Study the drawing (mm; zero at the part's minimum x, y, z) and answer. Coordinates: 2 decimals unless noted, no trailing zeros. Order: outer loops, then holes, each group sorted by start corner. A loop starts at its lowest first (then second) coordinate and runs counter-clockwise, first axis right, second up.
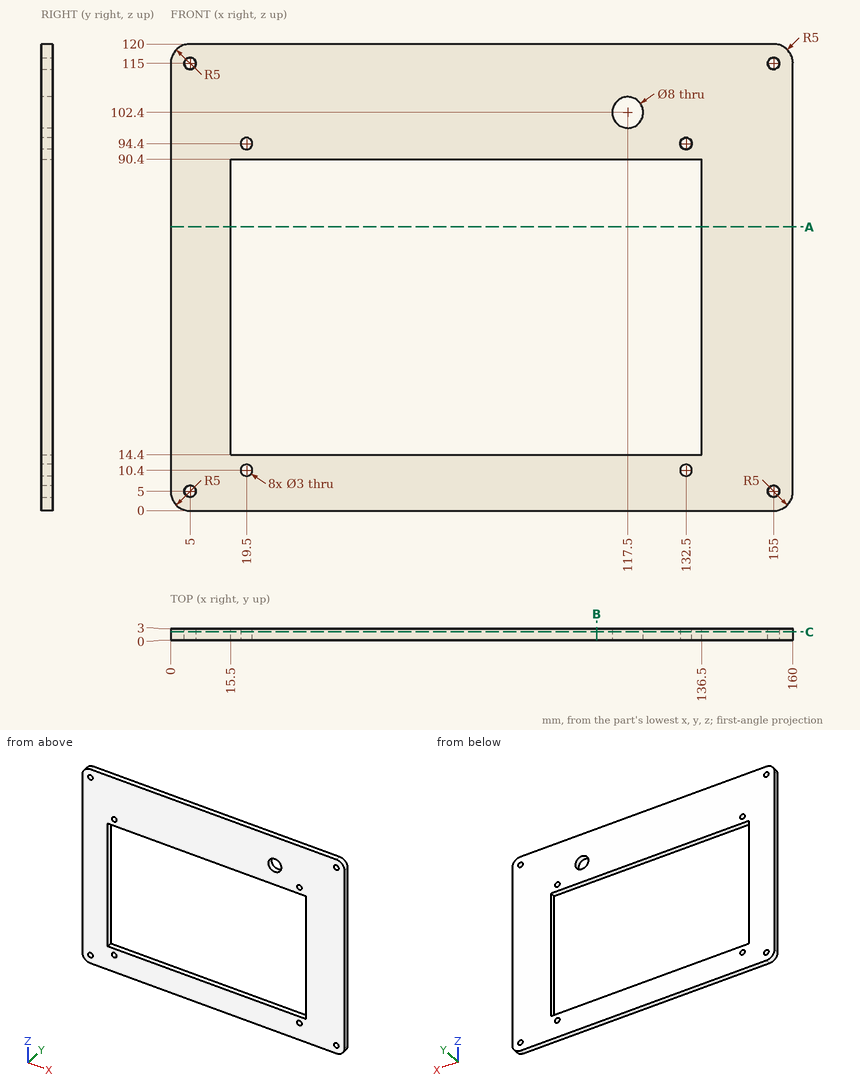
1) A cutting plane is placed at A-A, the plane z = 73. Determine the outline of the cut face in (x, y), and give its area (3 significant figures).
A:
outline: (0, 0) - (15.5, 0) - (15.5, 3) - (0, 3) - close; (136.5, 0) - (160, 0) - (160, 3) - (136.5, 3) - close
area: 117 mm2
2) A cutting plane is placed at C-C, the plane y = 2.2. State how many separate pieces and enclosed holes the cut face has, and give its area (3 significant figures).
A:
separate pieces: 1
enclosed holes: 10
area: 9,880 mm2
3) Straight lines are drawn through the part: line 1 (Z direction, x = 19.5, y = 0.8); line 2 (X direction, y = 1, z = 5); line 3 (Z direction, x = 35, y = 2.05). For each, find the intervals that lie inside material, in ascending order.
A:
line 1: z = 0 to 8.9, 11.9 to 14.4, 90.4 to 92.9, 95.9 to 120
line 2: x = 0 to 3.5, 6.5 to 153.5, 156.5 to 160
line 3: z = 0 to 14.4, 90.4 to 120
4) A cutting plane is placed at B-B, the plane x = 109.5. Determine the outline of the cut face in (y, z).
A:
outline: (0, 0) - (3, 0) - (3, 14.4) - (0, 14.4) - close; (0, 90.4) - (3, 90.4) - (3, 120) - (0, 120) - close
